```python
from build123d import *

# Parameters (mm, degrees)
SKETCH1_W           = 10.1
SKETCH1_H           = 80
BOSS_EXTRUDE1_DEPTH = 20
CUT_EXTRUDE1_REACH  = 85.078
SKETCH2_R           = 6
FILLET1_R           = 5
SKETCH3_R           = 4
BOSS_EXTRUDE2_DEPTH = 8.5
SKETCH4_R           = 5.65
BOSS_EXTRUDE3_DEPTH = 1.5


with BuildPart() as part:
    # Sketch1 → Boss-Extrude1 (new body)
    with BuildSketch(Plane(origin=(0, 0, 0), x_dir=(1, 0, 0), z_dir=(0, 1, 0))):
        with Locations((5.05, 40)):
            Rectangle(SKETCH1_W, SKETCH1_H)
    extrude(amount=BOSS_EXTRUDE1_DEPTH)

    # Sketch2 → Cut-Extrude1 (cut, up to next)
    with BuildSketch(Plane(origin=(10.1, 0, 0), x_dir=(0, 0, -1), z_dir=(1, 0, 0)), mode=Mode.PRIVATE) as cut_extrude1_sk1:
        with Locations((10, 10)):
            Circle(SKETCH2_R)
    cut_extrude1_tool1 = extrude(cut_extrude1_sk1.sketch, amount=-CUT_EXTRUDE1_REACH, mode=Mode.PRIVATE) & part.part
    add(cut_extrude1_tool1.solids().sort_by_distance((10.1, 10, -10))[0], mode=Mode.SUBTRACT)

    # Fillet1
    fillet1_edges = [part.edges().sort_by_distance(p)[0] for p in [
        (5.05, 0, 0),
        (5.05, 20, 0),
    ]]
    fillet(fillet1_edges, radius=FILLET1_R)

    # Sketch3 → Boss-Extrude2 (add)
    with BuildSketch(Plane(origin=(0, 0, -80), x_dir=(-1, 0, 0), z_dir=(0, 0, -1))):
        with Locations(Location((-5.05, 10, 0), (0, 0, 180))):
            Circle(SKETCH3_R)
    extrude(amount=BOSS_EXTRUDE2_DEPTH)

    # Sketch4 → Boss-Extrude3 (add)
    with BuildSketch(Plane(origin=(0, 0, -80), x_dir=(-1, 0, 0), z_dir=(0, 0, -1))):
        with Locations(Location((-5.05, 10, 0), (0, 0, 206.64461444))):
            Circle(SKETCH4_R)
    extrude(amount=BOSS_EXTRUDE3_DEPTH)


solid = part.part
```
Input: part model. Units: mm. Frame: model coordinates. A direction names the side the tool comes from. Round coordinates to 2 decimals unless told otherwise and drop trailing zeros. Loops run counter-clockwise (first coordinate to the right, second up) from the corner with the lowest first, then second, coordinate; pieces in that order, holes last. Notation, with made-up numbers: M 49.25,-5 L 53.25,-5 A4 cw 53.25,-1 Z; hole C 2.5,79 d9. An arc over 180 degrees is marked long. Answer in a Markdown table with one row per item. Add a question column.
1. Set-up query: faces 4 (the face through (5, 0, -43)), 5 (the face through (0, 10, -39)), 6 (the face through (8.745, 11.532, -84.951)). Return all of +Z, -Z, +X, -X, +Y, -Y with unobstructed straight access to the full face (end or side cutting, diameter ignored); none if empty.
2. Section B-B (z = -10). Output: boundary loops of the cut face in (x, y).
3. Section D-D (y = 1.75). Output: boundary loops of the cut face in (x, z), and give its area (3 significant figures).
4. Section A-A (y = 10). Output: boundary loops of the cut face in (x, z).
5. Ray query, probe 1 along Y at (x, z) = (7, -10); probe 2 along X at (y, z) = (14.75, -70.5); probe 3 along Z at (x, y) = (8, 5.5). Return the intervals inside material, ascending.
6. Section C-C (x = 5.05). Output: boundary loops of the cut face in (y, z), and give its area (3 significant figures).
7. Contact query for flat-ended pins moving along their axis: pin 1 (1.5 mm diameter, centred on y = 15.5, z = -35, fed in from -X); pin 2 (6 mm diameter, centred on x = 3, y = 3, fed in from -Z); pin 3 (0.5 mm diameter, centred on x = 10.5, y = 9.5, fed in from +Z). Output: stop coordinate, or through.
8. Mould query, pull axis Z, two halves, no side actions, for faces 1 (the face through (2, 13, -81.5)), 2 (the face through (5.121, 4.143, -8.699)), 3 (the face through (10.1, 10, -39)). Classes: released by +Z, released by -Z, zero draft, split by the parting line, or undercut.
Values follow:
| question | item | result |
|---|---|---|
| 1 | face 4 | +Z, -Z, +X, -X, -Y |
| 1 | face 5 | +Z, -X, +Y, -Y |
| 1 | face 6 | -Z |
| 2 | outline | M 0,0 L 10.1,0 L 10.1,4 L 0,4 Z; M 0,16 L 10.1,16 L 10.1,20 L 0,20 Z |
| 3 | outline | M 0,-80 L 10.1,-80 L 10.1,-1.2 L 0,-1.2 Z |
| 3 | area | 796 mm^2 |
| 4 | outline | M -0.6,-81.5 L 1.05,-81.5 L 1.05,-88.5 L 9.05,-88.5 L 9.05,-81.5 L 10.7,-81.5 L 10.7,-80 L 10.1,-80 L 10.1,-16 L 0,-16 L 0,-80 L -0.6,-80 Z; M 0,-4 L 10.1,-4 L 10.1,0 L 0,0 Z |
| 5 | probe 1 | 0 to 4, 16 to 20 |
| 5 | probe 2 | 0 to 10.1 |
| 5 | probe 3 | -81.5 to -13.97, -6.03 to 0 |
| 6 | outline | M 0,-80 L 4.35,-80 L 4.35,-81.5 L 6,-81.5 L 6,-88.5 L 14,-88.5 L 14,-81.5 L 15.65,-81.5 L 15.65,-80 L 20,-80 L 20,-5 A5 ccw 15,0 L 5,0 A5 ccw 0,-5 Z; hole C 10,-10 d12 |
| 6 | area | 1,550 mm^2 |
| 7 | pin 1 | x = 0 |
| 7 | pin 2 | z = -81.5 |
| 7 | pin 3 | z = -80 |
| 8 | face 1 | released by -Z |
| 8 | face 2 | undercut |
| 8 | face 3 | zero draft |
